Here's how the part is built. I have some questions about the finished solid (model axes, mm). Face numbers are marked on the shaded views. A direction names the side the tool comes from. Coordinates: 2 decimals unless noted, no trailing zeros. Write each loop counter-clockwise with the first axis right and the second up, starting at its lowest first coordinate (ties: lowest second). Pieces come first, ordered by that corner, then holes.
Item 1: For the marked faces 4, 5 and 6, which set-ups out of +Z, -Z, +X, -X, +Y, -Y let a thin tool reach every point of the face, with its end or its side?
Item 2: If we section it at D-D (z = -2.5): Please give me the cut outline in (x, y).
Item 3: If we section it at C-C (y = 10): Please give me the cut outline in (x, z) (3 decimals), then the cut area to 3 significant figures.
Item 4: If we section it at B-B (x = 3.25): Please give me the cut outline in (y, z) (3 decimals), then the cut area to 3 significant figures.
Item 5: We'd pull the mould along X, two halves only. Please class the marked faces 1, 2 and 3: +X half, -X half, draft (parallel to the pull), parting line (faces both ways), or undercut.
Item 6: If we section it at A-A (x = 0.5): Please give me the cut outline in (y, z) (3 decimals), then the cut area to 3 significant figures.
Item 7: I'm going to push flat-ended pins straight in: pin 1 Ø6 at (y, z) = (6, 5) entering from +X; pin 2 Ø1.3 at (y, z) = (8.5, 1) entering from -X. Where does each tip first touch, or does it pass through?
Item 8: If I drill on line 1 (Z direction, x = 0.25, y = 8.5) (3 decimals); line 2 (X direction, y = 16, z = -0.75); line 3 (Z direction, x = 3.5, y = 13.5) (3 decimals), over which ranges is the centre line in solid material (lowest first)?
from build123d import *

# Parameters (mm, degrees)
SKETCH1_W           = 2.03
SKETCH1_H           = 4.03
BOSS_EXTRUDE1_DEPTH = 24
SKETCH2_W           = 1
SKETCH2_H           = 24
CUT_EXTRUDE1_DEPTH  = 2
SKETCH3_R           = 1.9
SKETCH3_R_2         = 0.9
BOSS_EXTRUDE2_DEPTH = 1
SKETCH4_R           = 1.15
CUT_EXTRUDE2_DEPTH  = 4


with BuildPart() as part:
    # Sketch1 → Boss-Extrude1 (new body)
    with BuildSketch(Plane(origin=(0, 0, 0), x_dir=(1, 0, 0), z_dir=(0, 1, 0))):
        Polygon((0.758759529, 5.315), (5, 5.315), (5, -7.215), (1.398203198, -7.215), (-1.03, -7.215), (-1.03, -1.785), (4, -1.785), (4, -0.115), (-1.03, -0.115), (-1.03, 5.315), align=None)
        with Locations((0.985, 2.3)):
            Rectangle(SKETCH1_W, SKETCH1_H, mode=Mode.SUBTRACT)
        with Locations((0.985, -4.2)):
            Rectangle(SKETCH1_W, SKETCH1_H, mode=Mode.SUBTRACT)
    extrude(amount=BOSS_EXTRUDE1_DEPTH)

    # Sketch2 → Cut-Extrude1 (cut)
    with BuildSketch(Plane.ZY.offset(1.03)):
        with Locations((-2.315, 12)):
            Rectangle(SKETCH2_W, SKETCH2_H)
        with Locations((4.215, 12)):
            Rectangle(SKETCH2_W, SKETCH2_H)
    extrude(amount=-CUT_EXTRUDE1_DEPTH, mode=Mode.SUBTRACT)

    # Sketch3 → Boss-Extrude2 (add)
    with BuildSketch(Plane(origin=(5, 0, 0), x_dir=(0, 0, -1), z_dir=(1, 0, 0))):
        with Locations((2.815, 19)):
            Circle(SKETCH3_R)
        with Locations((2.815, 19)):
            Circle(SKETCH3_R_2, mode=Mode.SUBTRACT)
        with Locations((2.815, 5)):
            Circle(SKETCH3_R)
        with Locations((2.815, 5)):
            Circle(SKETCH3_R_2, mode=Mode.SUBTRACT)
    extrude(amount=BOSS_EXTRUDE2_DEPTH)

    # Sketch4 → Cut-Extrude2 (cut)
    with BuildSketch(Plane(origin=(5, 0, 0), x_dir=(0, 0, -1), z_dir=(1, 0, 0))):
        with Locations((2.815, 19)):
            Circle(SKETCH4_R)
        with Locations((2.815, 5)):
            Circle(SKETCH4_R)
    extrude(amount=-CUT_EXTRUDE2_DEPTH, mode=Mode.SUBTRACT)


solid = part.part
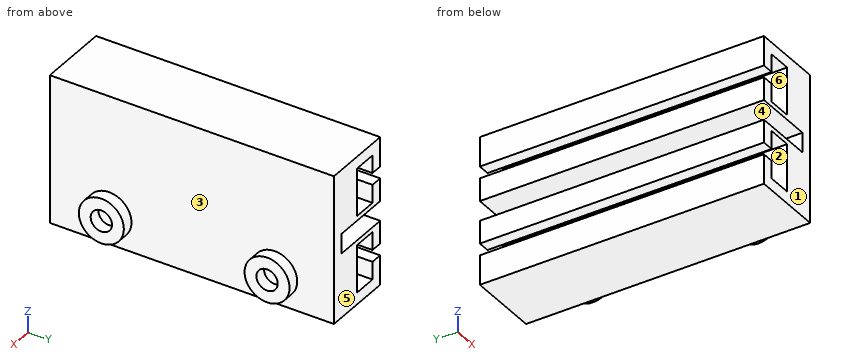
Answer list:
1. face 4: -X, +Y, -Y
1. face 5: +Z, -Z, +X, -X, +Y
1. face 6: +Y, -Y
2. outline: (2, 0) - (5, 0) - (5, 3.13) - (6, 3.13) - (6, 4.16) - (5, 4.16) - (5, 3.89) - (2, 3.89) - close; (2, 6.11) - (5, 6.11) - (5, 5.84) - (6, 5.84) - (6, 6.87) - (5, 6.87) - (5, 17.13) - (6, 17.13) - (6, 18.16) - (5, 18.16) - (5, 17.89) - (2, 17.89) - close; (2, 20.11) - (5, 20.11) - (5, 19.84) - (6, 19.84) - (6, 20.87) - (5, 20.87) - (5, 24) - (2, 24) - close
3. outline: (-1.03, -5.315) - (5, -5.315) - (5, 7.215) - (-1.03, 7.215) - (-1.03, 4.715) - (-0.03, 4.715) - (-0.03, 6.215) - (2, 6.215) - (2, 2.185) - (-0.03, 2.185) - (-0.03, 3.715) - (-1.03, 3.715) - (-1.03, 1.785) - (4, 1.785) - (4, 0.115) - (-1.03, 0.115) - (-1.03, -1.815) - (-0.03, -1.815) - (-0.03, -0.285) - (2, -0.285) - (2, -4.315) - (-0.03, -4.315) - (-0.03, -2.815) - (-1.03, -2.815) - close
3. area: 48.8 mm2
4. outline: (0, -5.315) - (24, -5.315) - (24, 0.115) - (0, 0.115) - close; (0, 1.785) - (24, 1.785) - (24, 7.215) - (0, 7.215) - close; hole circle Ø2.3 at (5, -2.815); hole circle Ø2.3 at (19, -2.815)
4. area: 252 mm2
5. face 1: draft
5. face 2: undercut
5. face 3: +X half
6. outline: (0, -5.315) - (24, -5.315) - (24, -4.315) - (0, -4.315) - close; (0, -0.285) - (24, -0.285) - (24, 0.115) - (0, 0.115) - close; (0, 1.785) - (24, 1.785) - (24, 2.185) - (0, 2.185) - close; (0, 6.215) - (24, 6.215) - (24, 7.215) - (0, 7.215) - close
6. area: 67.2 mm2
7. pin 1: stops at x = 5
7. pin 2: stops at x = 4
8. line 1: z = -5.315 to -4.315, -0.285 to 0.115, 1.785 to 2.185, 6.215 to 7.215
8. line 2: x = -1.03 to -0.03, 2 to 5
8. line 3: z = -5.315 to 0.115, 1.785 to 7.215
